Input: dimensioned drawing with shaded views. Units: mm. Origin: part minimum x, y, z. Round coordinates to 2 decimals unless told otherwise and drop trailing zeros. Loops run counter-clockwise (first coordinate to the right, second up) from the corner with the lowest first, then second, coordinate; pieces in that order, holes last. Notation, with made-up numbers: (70, 0.25) - (126, 0.25) arc R33 ccw to (126, 32.25) - close; hole circle Ø1 at (-7, 49.5). An arc over 180 degrees is marked (long way). One line per question, with ' | ' between items. Start each with the question number.
Item 1: Section B-B, the plane y = 1.7. Give the number of separate pieces and of enclosed holes in the cut face, plus the area to 3 significant figures.
Item 2: Material intervals for line 1 along X through (y, z) = (2.05, 36.5); line 2 along X through (y, z) = (1.85, 54.5); line 3 along Z through (x, y) = (91.5, 2.2), sorted ascending.
Item 3: Section A-A, the plane x = 97.5. Return loops of the section in (y, z), plus the area to 3 significant figures.
Item 4: Section C-C, the plane x = 60. Return loops of the section in (y, z).
Item 5: First-contact query: pin 1 (2.5 mm diameter, centred on x = 45, z = 5.5, fed in from -Y). Flat tip, straight axial feed; report the tip coordinate or a pass-through.
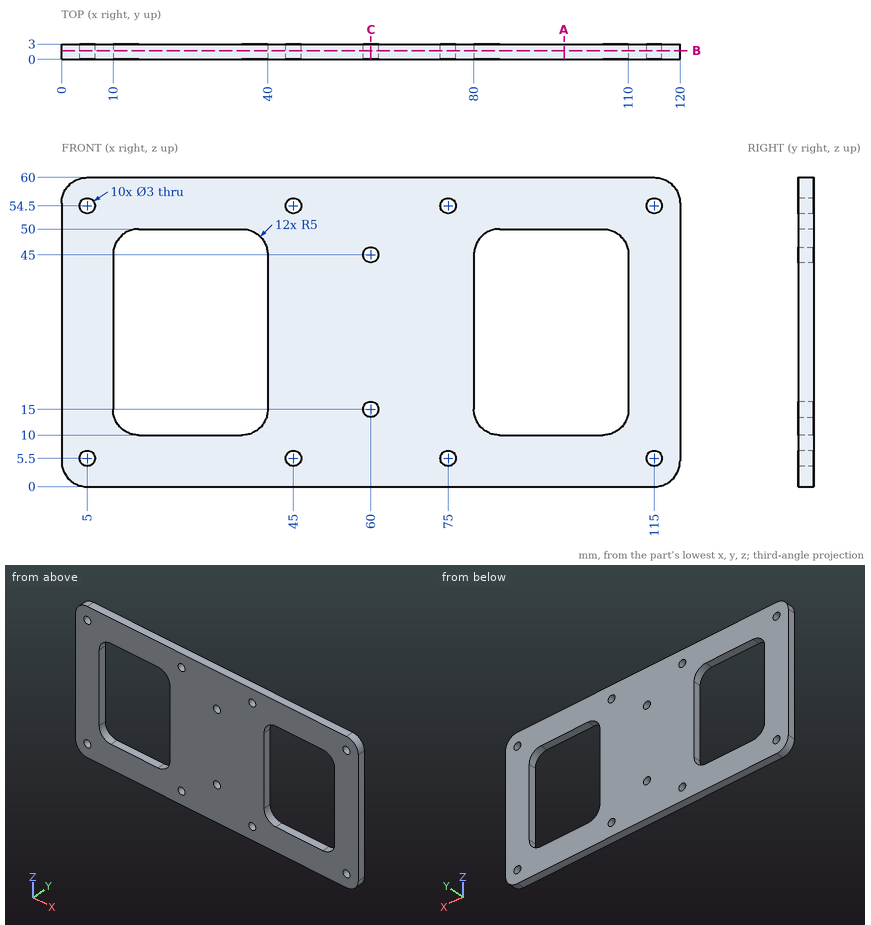
Return value:
1) separate pieces: 1 | enclosed holes: 12 | area: 4,750 mm2
2) line 1: 0 to 10, 40 to 80, 110 to 120 | line 2: 0 to 3.5, 6.5 to 43.5, 46.5 to 73.5, 76.5 to 113.5, 116.5 to 120 | line 3: 0 to 10, 50 to 60
3) outline: (0, 0) - (3, 0) - (3, 10) - (0, 10) - close; (0, 50) - (3, 50) - (3, 60) - (0, 60) - close | area: 60.0 mm2
4) outline: (0, 0) - (3, 0) - (3, 13.5) - (0, 13.5) - close; (0, 16.5) - (3, 16.5) - (3, 43.5) - (0, 43.5) - close; (0, 46.5) - (3, 46.5) - (3, 60) - (0, 60) - close
5) pin 1: through
